Build history of the part. All positions in model axes, mm. A direction names the side the tool comes from. Give positions to 0.01 mm unless a question says otherwise; leave off trailing zeros. Write each loop counter-clockwise with the first axis right and the second up, starting at its lowest first coordinate (ties: lowest second). Pieces come first, ordered by that corner, then holes. Notation, with made-up numbers: M 11,17.25 L 28,17.25 A15 cw 28,43.25 Z; hole C 76,79.5 d6. An arc over 180 degrees is marked long. Return JSON: item names as keys, results as strings. Group by question number.
Q1. Band-saw the part on B-B, the plane y = 63.5. Give the cut face in (x, z), then the cut area to 3 significant figures.
Q2. Flat gauge pins, fed straight in: pin 1 Ø1.8 at (x, z) = (147, -0.025) entering from -Y; pin 2 Ø1.8 at (y, z) = (25, 70) entering from -X. Where does each tip first touch, or does it go through?
Q3. Wall check: probe 1 along Z at (x, y) = (147, 9.75) (3 decimals); probe 2 along Y at (x, z) = (146.2, 69.5); probe 3 along Y at (x, z) = (147.6, -69.5). Give the ranges that are in metal, low to high.
Q4. Tool access for faces 4 (the flat face through (147, 16, -40)), 5 (the cylindrical face through (148.479, 23.981, 71.026)), 6 (the flat face through (147, 22, -68)): list every direction of +Z, -Z, +X, -X, +Y, -Y with a clear straight run to the whole face (end or side of a thin tool).
Q5. Band-saw the part on A-A, the plane y = 13.5. Give the cut face in (x, z) (3 decimals), then the cut area to 3 significant figures.
Q6. Pull direction Z, two halves, no side cores. Call faces 1 (the flat face through (147, 62, -68)), 2 (the flat face through (147, 43, 72.5)), 3 (the flat face through (147, 43, -72.5)): +Z half, -Z half, draft (parallel to the pull), parting line (faces both ways), or undercut.
from build123d import *

# Parameters (mm, degrees)
SKETCH_1_W          = 300
SKETCH_1_H          = 145
EXTRUDE_1_DEPTH     = 81
SHELL_1_T           = -6
SKETCH_2_R          = 2.55
CUT_EXTRUDE_1_DEPTH = 183.705363906
SKETCH_3_R          = 4.25
CUT_EXTRUDE_2_DEPTH = 3
SKETCH_4_W          = 145
SKETCH_4_H          = 81
CUT_EXTRUDE_3_DEPTH = 314.453744594
SKETCH_5_W          = 145
SKETCH_5_H          = 6
CUT_EXTRUDE_4_DEPTH = 109.872632006
SKETCH_6_R          = 1.6
SKETCH_6_R_2        = 1.25
CUT_EXTRUDE_5_DEPTH = 109.872632006
SKETCH_7_R          = 2.95
CUT_EXTRUDE_6_DEPTH = 3
SKETCH_8_R          = 1.5
CUT_EXTRUDE_7_DEPTH = 10


with BuildPart() as part:
    # ｽｹｯﾁ1 → ﾎﾞｽ - 押し出し1 (new body)
    with BuildSketch(Plane(origin=(0, 0, 0), x_dir=(1, 0, 0), z_dir=(0, 1, 0))):
        Rectangle(SKETCH_1_W, SKETCH_1_H)
    extrude(amount=EXTRUDE_1_DEPTH)

    # ｼｪﾙ1
    shell_1_openings = [part.faces().sort_by_distance(p)[0] for p in [
        (0, 81, 0),
    ]]
    offset(amount=SHELL_1_T, openings=shell_1_openings, kind=Kind.INTERSECTION)

    # ｽｹｯﾁ2 → ｶｯﾄ - 押し出し1 (cut, through all)
    with BuildSketch(Plane(origin=(0, 6, 0), x_dir=(1, 0, 0), z_dir=(0, 1, 0))):
        with Locations(Location((140, 60, 0), (0, 0, 270))):
            Circle(SKETCH_2_R)
        with Locations(Location((140, -60, 0), (0, 0, 90))):
            Circle(SKETCH_2_R)
        with Locations(Location((-22.5, -60, 0), (0, 0, 270))):
            Circle(SKETCH_2_R)
        with Locations(Location((-22.5, 60, 0), (0, 0, 90))):
            Circle(SKETCH_2_R)
    extrude(amount=-CUT_EXTRUDE_1_DEPTH, mode=Mode.SUBTRACT)

    # ｽｹｯﾁ3 → ｶｯﾄ - 押し出し2 (cut)
    with BuildSketch(Plane(origin=(0, 6, 0), x_dir=(1, 0, 0), z_dir=(0, 1, 0))):
        with Locations(Location((140, 60, 0), (0, 0, 270))):
            Circle(SKETCH_3_R)
        with Locations(Location((-22.5, 60, 0), (0, 0, 270))):
            Circle(SKETCH_3_R)
        with Locations(Location((-22.5, -60, 0), (0, 0, 270))):
            Circle(SKETCH_3_R)
        with Locations(Location((140, -60, 0), (0, 0, 270))):
            Circle(SKETCH_3_R)
    extrude(amount=-CUT_EXTRUDE_2_DEPTH, mode=Mode.SUBTRACT)

    # ｽｹｯﾁ4 → ｶｯﾄ - 押し出し3 (cut, through all)
    with BuildSketch(Plane.ZY.offset(-144)):
        with Locations((0, 40.5)):
            Rectangle(SKETCH_4_W, SKETCH_4_H)
    extrude(amount=CUT_EXTRUDE_3_DEPTH, mode=Mode.SUBTRACT)

    # ｽｹｯﾁ5 → ｶｯﾄ - 押し出し4 (cut, through all)
    with BuildSketch(Plane.ZY.offset(-144)):
        with Locations((0, 3)):
            Rectangle(SKETCH_5_W, SKETCH_5_H)
    extrude(amount=-CUT_EXTRUDE_4_DEPTH, mode=Mode.SUBTRACT)

    # ｽｹｯﾁ6 → ｶｯﾄ - 押し出し5 (cut, through all)
    with BuildSketch(Plane.ZY.offset(-144)):
        with Locations((-69.5, 63.5)):
            Circle(SKETCH_6_R)
        with Locations(Location((-69.5, 23.5, 0), (0, 0, 180))):
            Circle(SKETCH_6_R)
        with Locations((69.5, 23.5)):
            Circle(SKETCH_6_R)
        with Locations(Location((69.5, 63.5, 0), (0, 0, 180))):
            Circle(SKETCH_6_R)
        with Locations((-40, 5.3)):
            Circle(SKETCH_6_R_2)
        with Locations((0, 5.3)):
            Circle(SKETCH_6_R_2)
        with Locations((40, 5.3)):
            Circle(SKETCH_6_R_2)
    extrude(amount=-CUT_EXTRUDE_5_DEPTH, mode=Mode.SUBTRACT)

    # ｽｹｯﾁ7 → ｶｯﾄ - 押し出し6 (cut)
    with BuildSketch(Plane.ZY.offset(-144)):
        with Locations((-69.5, 63.5)):
            Circle(SKETCH_7_R)
        with Locations((-69.5, 23.5)):
            Circle(SKETCH_7_R)
        with Locations((69.5, 63.5)):
            Circle(SKETCH_7_R)
        with Locations((69.5, 23.5)):
            Circle(SKETCH_7_R)
    extrude(amount=-CUT_EXTRUDE_6_DEPTH, mode=Mode.SUBTRACT)

    # ｽｹｯﾁ8 → ｶｯﾄ - 押し出し7 (cut)
    with BuildSketch(Plane.XZ.offset(-6)):
        with Locations(Location((147, 40, 0), (0, 0, 270))):
            Circle(SKETCH_8_R)
        with Locations(Location((147, -0.025, 0), (0, 0, 270))):
            Circle(SKETCH_8_R)
        with Locations(Location((147, -40, 0), (0, 0, 270))):
            Circle(SKETCH_8_R)
    extrude(amount=-CUT_EXTRUDE_7_DEPTH, mode=Mode.SUBTRACT)


solid = part.part
From the geometry:
{
 "1": {"outline": "M 144,-72.5 L 150,-72.5 L 150,-71.1 L 147,-71.1 L 147,-72.45 L 144,-72.45 Z; M 144,-66.55 L 147,-66.55 L 147,-67.9 L 150,-67.9 L 150,67.9 L 147,67.9 L 147,66.55 L 144,66.55 Z; M 144,72.45 L 147,72.45 L 147,71.1 L 150,71.1 L 150,72.5 L 144,72.5 Z", "area": "815 mm^2"},
 "2": {"pin 1": "stops at y = 16", "pin 2": "stops at x = 147"},
 "3": {"probe 1": "z = -72.5 to -41.5, -38.5 to -1.525, 1.475 to 38.5, 41.5 to 72.5", "probe 2": "y = 6 to 20.55, 26.45 to 60.55, 66.45 to 81", "probe 3": "y = 6 to 21.9, 25.1 to 61.9, 65.1 to 81"},
 "4": {"face 4": "-Y", "face 5": "+X, -X", "face 6": "-X"},
 "5": {"outline": "M 144,-72.5 L 150,-72.5 L 150,72.5 L 144,72.5 Z; hole C 147,-40 d3; hole C 147,-0.025 d3; hole C 147,40 d3", "area": "849 mm^2"},
 "6": {"face 1": "undercut", "face 2": "+Z half", "face 3": "-Z half"}
}
